Source: CAD feature listing. Evaluate the final solid. Frame: model axes, mm. Coordinates: 2 decimals unless noted, no trailing zeros. Order: outer loops, then holes, each group sorted by start corner. A loop starts at its lowest first (then second) coordinate and runs counter-clockwise, first axis right, second up.
Item 1: Section B-B on y = 0.15. Return the cut outline in (x, z), then the cut area to 3 significant figures.
Item 2: Mould query, pull axis Z, two halves, no side actions, for faces 1 (the cylindrical face through (-0.69, 0, 24.48)), 2 (the cylindrical face through (-4.57, 0, -10.5)), 3 (the cylindrical face through (-0.65, 0, -24.43)). Classes: released by +Z, released by -Z, zero draft, split by the parting line, or undercut.
Item 3: Ray query, line 1 (X direction, y = -0.1, z = 9); line 2 (Z direction, x = -4.5, y = 0.05); line 3 (Z direction, x = -24, y = 0.05). Return the intervals inside material, ascending.
Item 4: Contact query for a flat-ended pin moving along its axis: P1, Ø2.5, axis at x = -4.5, z = 9, coming from the -Y side. Output: stop coordinate, or through.
Item 5: Section D-D on x = -19. Return the cut outline in (y, z).
Item 6: Section C-C on x = -4.5. Return the cut outline in (y, z).
Item 7: Section A-A on z = -9. Return the cut outline in (x, y), then the cut area to 3 significant figures.
Autodesk Inventor part; units mm, degrees
ref_plane "YZ Plane" through (0, 0, 0) normal (1, 0, 0) x (0, 1, 0)
ref_plane "XZ Plane" through (0, 0, 0) normal (0, 1, 0) x (-1, 0, 0)
ref_plane "XY Plane" through (0, 0, 0) normal (0, 0, 1) x (1, 0, 0)
sketch "Skizze1" plane through (0, 0, 0) normal (0, 1, 0) x (-1, 0, 0)
  line L0 (0, 25) -> (0, -25)
  line L1 (0, 25) -> (95, 45)
  line L2 (95, 45) -> (95, -45)
  line L3 (95, -45) -> (0, -25)
  point P0 (0, 0)
  point P1 (0, 0)
  dimension "d0" = 90
  dimension "d1" = 95
  dimension "d2" = 50
extrude "Grobblech1" add sketch "Skizze1" along normal mid plane 0.5
sketch "Skizze3" plane through (0, 0.25, 0) normal (0, 1, 0) x (1, 0, 0)
  line L0 (0, 25) -> (0, -25)
  point P0 (0, 0)
  point P1 (-4.5, -9)
  point P2 (-4.5, 9)
  dimension "d16" = 16
  dimension "d17" = 16
  dimension "d18" = 4.5
  dimension "d19" = 4.5
hole "Bohrung2" at (-4.5, 0.25, 9) at (-4.5, 0.25, -9) direction (0, -1, 0) diameter 3 end through all
fillet "Rundung1" radius 7 2 edges at (-95, 0, -45) (-95, 0, 45)
fillet "Rundung2" radius 3 2 edges at (0, 0, -25) (0, 0, 25)
equation "\"d3\" = Stärke"
equation "\"Biegeradius\" = Stärke"
equation "\"BreiteBiegungsfreistellung\" = Stärke"
equation "\"TiefeBiegungsfreistellung\" = 0.5 * Stärke"
equation "\"GrößeEckenfreistellung\" = 4 * Stärke"
equation "\"MinimalRest\" = 2 * Stärke"
equation "\"Übergangsradius\" = Biegeradius"
equation "\"JacobiRadiusGröße\" = Biegeradius"
equation "\"Abstandsgröße\" = Stärke"
properties part number "propeller_extensions" material "Glas"
Answer list:
1. outline: (-95, -36.37) arc R7 ccw to (-86.56, -43.22) - (-2.38, -25.5) arc R3 ccw to (0, -22.57) - (0, 22.57) arc R3 ccw to (-2.38, 25.5) - (-86.56, 43.22) arc R7 ccw to (-95, 36.37) - close; hole circle Ø3 at (-4.5, -9); hole circle Ø3 at (-4.5, 9)
1. area: 6,600 mm2
2. face 1: released by +Z
2. face 2: undercut
2. face 3: released by -Z
3. line 1: x = -95 to -6, -3 to 0
3. line 2: z = -25.95 to -10.5, -7.5 to 7.5, 10.5 to 25.95
3. line 3: z = -30.05 to 30.05
4. P1: passes through
5. outline: (-0.25, -29) - (0.25, -29) - (0.25, 29) - (-0.25, 29) - close
6. outline: (-0.25, -25.95) - (0.25, -25.95) - (0.25, -10.5) - (-0.25, -10.5) - close; (-0.25, -7.5) - (0.25, -7.5) - (0.25, 7.5) - (-0.25, 7.5) - close; (-0.25, 10.5) - (0.25, 10.5) - (0.25, 25.95) - (-0.25, 25.95) - close
7. outline: (-95, -0.25) - (-6, -0.25) - (-6, 0.25) - (-95, 0.25) - close; (-3, -0.25) - (0, -0.25) - (0, 0.25) - (-3, 0.25) - close
7. area: 46.0 mm2
